Part print with two shaded views. Sizes in mm from the minimum x, y, z corner. Round coordinates to 2 decimals unless told otherwise and drop trailing zeros. Write each loop counter-clockwise with the first axis right and the second up, starting at its lowest first coordinate (ties: lowest second). Pieces come first, ordered by that corner, then holes. Notation, with made-up numbers: (60, 36) - (93, 36) arc R15 ccw to (93, 48) - close; hole circle Ø6 at (67, 31.25). An arc over 180 degrees is marked (long way). Use one line per item in the form item = value. Start each with the question number.
Item 1: Drill centre lines: L1, parallel to Y at x = 57.5, z = 2.65; L2, parallel to Y at x = 31.75, z = 2.35 (1 decimal). Where is each one in solid material? Low to high.
Item 2: Band-saw the part on A-A, the plane x = 57.15. List the corners of the cut face in (y, z), and give its area (3 significant figures).
Item 3: Band-saw the part on D-D, the plane x = 79.5. List the corners of the cut face in (y, z), and give its area (3 significant figures).
Item 4: Band-saw the part on C-C, the plane y = 31.75. List the corners of the cut face in (x, z) (1 decimal).
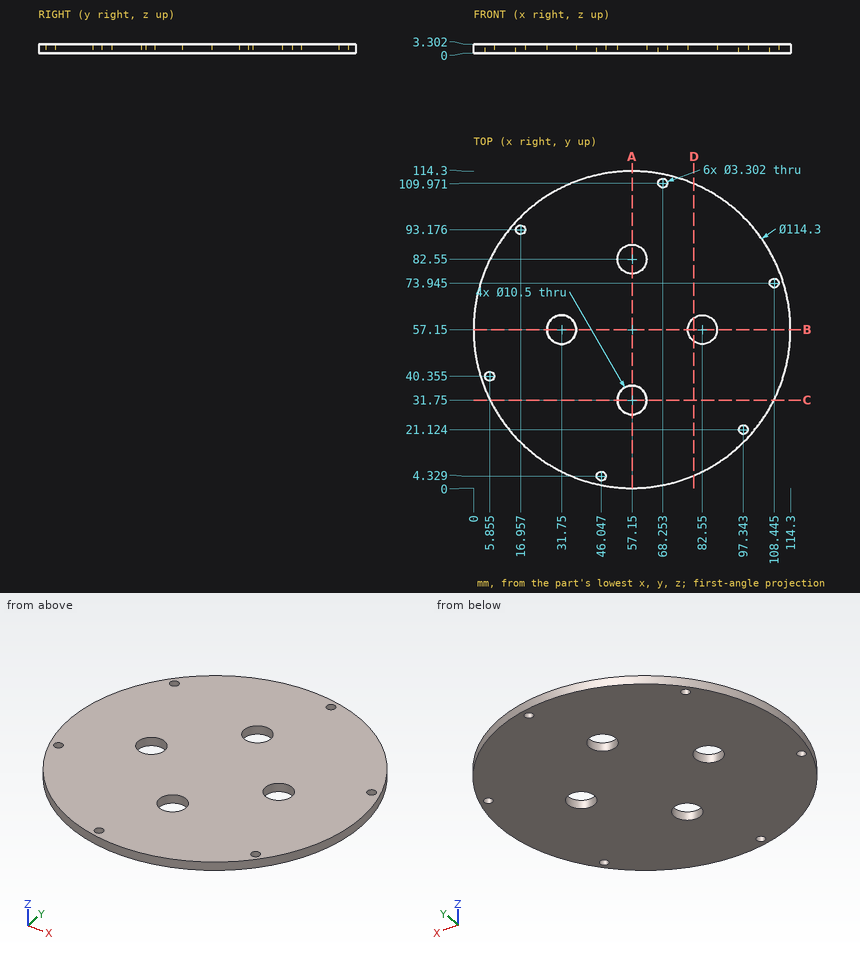
Determined:
q1.L1 = 0 to 26.51, 36.99 to 77.31, 87.79 to 114.3
q1.L2 = 6 to 51.9, 62.4 to 108.3
q2.outline = (0, 0) - (26.5, 0) - (26.5, 3.3) - (0, 3.3) - close; (37, 0) - (77.3, 0) - (77.3, 3.3) - (37, 3.3) - close; (87.8, 0) - (114.3, 0) - (114.3, 3.3) - (87.8, 3.3) - close
q2.area = 308 mm²
q3.outline = (4.55, 0) - (52.88, 0) - (52.88, 3.3) - (4.55, 3.3) - close; (61.42, 0) - (109.75, 0) - (109.75, 3.3) - (61.42, 3.3) - close
q3.area = 319 mm²
q4.outline = (6, 0) - (51.9, 0) - (51.9, 3.3) - (6, 3.3) - close; (62.4, 0) - (108.3, 0) - (108.3, 3.3) - (62.4, 3.3) - close
